Design review of the part built by this model. Coordinates are the model's own, in mm. A direction names the side the tool comes from. Give positions to 0.01 mm unless a question says otherwise; leave off trailing zeros. Loops run counter-clockwise (first coordinate to the right, second up) from the corner with the lowest first, then second, coordinate; pieces in that order, holes last. Notation, with made-up numbers: (37.25, 61.5) -> (87.25, 61.5) arc R33 cw to (87.25, 90.5) -> close; hole circle Ø7 at (86.25, -13.75). An arc over 180 degrees is marked (long way). Use a Markdown table: item, result. Add a question column.
1. For pin 1 Ø12 at (x, y) = (-92.5, 55.5) entering from -Z; pin 2 Ø11 at (y, z) = (56.5, 20) entering from -X; pin 3 Ø10 at (x, z) = (-135, 12.5) entering from +Y; pin 4 Ø3.5 at (x, z) = (-165.5, 38) entering from -Y, all flat-tipped, find the tip position at first contact; note any pin that passes through.
2. For faces 1 (the flat face through (-128.08, 5.65, 1.48)), 2 (the flat face through (-78.222, 44, 2)), 3 (the flat face through (-168, 16.67, 38)), 4 (the flat face through (-178.222, 54, 20)), 5 (the flat face through (-128, 53.67, 20)), list the 3-axis set-ups (+Z, -Z, +X, -X, +Y, -Y) from which the entire face can be reached by the end or side of a thin tool; tool diameter is ignored.
3. Add section A-A (y = 13). State the section outline as (x, z) points, and give its area (3 significant figures).
4. Add section B-B (y = 48.5). State the section outline as (x, z) points, and give its area (3 significant figures).
5. Add section D-D (x = -165). State the section outline as (y, z) points.
6. To check wall thickness, follow line 1 (Z direction, x = -99, y = 29); line 2 (Y direction, x = -147, z = 8); line 3 (X direction, y = 30, z = 38). State the ranges of each line that lie inside material, in increasing order.
7. Draft analysis for pull direction Z (two halves, no side actions). For faces 6 (the flat face through (-124, 38, 0)), 7 (the flat face through (-129, 62, 3)), 8 (the flat face through (-135, 39, 40)), 9 (the flat face through (-88.08, 5.65, 38.48)), state which applies: pulls with the +Z half, pulls with the -Z half, needs draft (parallel to the pull), parting line crosses it, or undercut.
8. Add section C-C (z = 12.5). State the section outline as (x, y) points.
```python
from build123d import *

# Parameters (mm, degrees)
F0_R      = 5
F1_DEPTH  = 40
F5_W      = 100
F5_H      = 3
F6_DEPTH  = 28
F7_W      = 100
F7_H      = 3
F8_DEPTH  = 10
F7_H_2    = 40
F13_DEPTH = 116.001
F14_W     = 100
F14_H     = 3
F15_DEPTH = 10
F18_DEPTH = 40.001
F19_SIZE  = 2
F20_SIZE  = 2
F21_W     = 67.4691606036
F21_H     = 7
F22_DEPTH = 116.001


with BuildPart() as f1:
    # F0 (on Top) → F1 (new body)
    with BuildSketch(Plane.XY):
        with BuildLine():
            Line((21.777506699, 52.6698508731), (21.777506699, 56.6698508731))
            Line((21.777506699, 56.6698508731), (-78.222493301, 56.6698508731))
            Line((-78.222493301, 56.6698508731), (-78.222493301, 16.6698508731))
            Line((-78.222493301, 16.6698508731), (-58.222493301, -5.6908289019))
            Line((-58.222493301, -5.6908289019), (-38.222493301, 16.6698508731))
            Line((-38.222493301, 16.6698508731), (-18.222493301, -5.6908289019))
            Line((-18.222493301, -5.6908289019), (1.777506699, 16.6698508731))
            Line((1.777506699, 16.6698508731), (21.777506699, 16.6698508731))
            Line((21.777506699, 16.6698508731), (31.377506699, 23.8698508731))
            ThreePointArc((31.377506699, 23.8698508731), (36.9564394679, 41.7294951294), (21.777506699, 52.6698508731))
        make_face()
        with Locations((21.777506699, 36.6698508731)):
            Circle(F0_R, mode=Mode.SUBTRACT)
    extrude(amount=F1_DEPTH)


with BuildPart() as f2_1:
    # F2: copy of F1
    add(f1.part.moved(Location((0, 0, 28))))


with BuildPart() as f4_1:
    # F4: copy of F1
    add(f1.part.moved(Location((0, 0, 34))))


with BuildPart() as f6:
    # F5 (on face) → F6 (new body)
    with BuildSketch(Plane.XY.offset(40)):
        with Locations((-28.222493301, 55.1698508731)):
            Rectangle(F5_W, F5_H)
    extrude(amount=F6_DEPTH)


with BuildPart() as f8:
    # F7 (on face) → F8 (new body)
    with BuildSketch(Plane(origin=(0, 56.6698508731, 0), x_dir=(-1, 0, 0), z_dir=(0, 1, 0))):
        with Locations((28.222493301, 69.5)):
            Rectangle(F7_W, F7_H)
    extrude(amount=F8_DEPTH)


with BuildPart() as f8b:
    # F7 (on face) → F8, piece 2 (new body)
    with BuildSketch(Plane(origin=(0, 56.6698508731, 0), x_dir=(-1, 0, 0), z_dir=(0, 1, 0))):
        with Locations((28.222493301, 20)):
            Rectangle(F7_W, F7_H_2)
    extrude(amount=F8_DEPTH)


with BuildPart() as f1_1:
    add(f1.part)

    # F12 (on face) → F13 (cut, through all)
    with BuildSketch(Plane(origin=(-78.222493301, 0, 0), x_dir=(0, -1, 0), z_dir=(-1, 0, 0))):
        Polygon((15.5293103307, 30), (-53.6698508731, 30), (-53.6698508731, 3), (13.7041052803, 3), align=None)
    extrude(amount=-F13_DEPTH, mode=Mode.SUBTRACT)

    # F14 (on face) → F15 (join)
    with BuildSketch(Plane(origin=(0, 56.6698508731, 0), x_dir=(-1, 0, 0), z_dir=(0, 1, 0))):
        with Locations((28.222493301, 1.5)):
            Rectangle(F14_W, F14_H)
        with Locations((28.222493301, 38.5)):
            Rectangle(F14_W, F14_H)
    extrude(amount=F15_DEPTH)

    # F16: F1 across face


with BuildPart() as f1_2:
    add(f1_1.part)
    add(f1_1.part.mirror(Plane(origin=(-78.222493301, 41.2061594964, 25.2897125567), x_dir=(0, -1, 0), z_dir=(-1, 0, 0))))

    # F17 (on face) → F18 (cut, through all)
    with BuildSketch(Plane.XY.offset(40)):
        Polygon((-78.222493301, 86.7001339793), (-78.222493301, 16.6698508731), (-78.222493301, -27.7220606804), (68.2113543153, -27.7220606804), (68.2113543153, 86.7001339793), align=None)
    extrude(amount=-F18_DEPTH, mode=Mode.SUBTRACT)

    # F19
    f19_edges = [f1_2.edges().sort_by_distance(p)[0] for p in [
        (-178.222493, 56.669851, 20),
    ]]
    chamfer(f19_edges, length=F19_SIZE)

    # F20
    f20_edges = [f1_2.edges().sort_by_distance(p)[0] for p in [
        (-78.222493, 56.669851, 20),
    ]]
    chamfer(f20_edges, length=F20_SIZE)

    # F21 (on face) → F22 (cut, through all)
    with BuildSketch(Plane.YZ.offset(-78.222493301)):
        with Locations((19.9352705713, 33.5)):
            Rectangle(F21_W, F21_H)
    extrude(amount=-F22_DEPTH, mode=Mode.SUBTRACT)


solid = f1_2.part
```
Taken from the geometry:
| question | item | result |
|---|---|---|
| 1 | pin 1 | stops at z = 0 |
| 1 | pin 2 | stops at x = -178.22 |
| 1 | pin 3 | stops at y = 56.67 |
| 1 | pin 4 | stops at y = 16.67 |
| 2 | face 1 | +Z, -Z, -Y |
| 2 | face 2 | +Z, -Z, +X, +Y, -Y |
| 2 | face 3 | +Z, -Z, -X, -Y |
| 2 | face 4 | +Z, -Z, -X, +Y |
| 2 | face 5 | +X, -X, -Y |
| 3 | outline | (-154.94, 0) -> (-121.5, 0) -> (-121.5, 3) -> (-154.94, 3) -> close; (-154.94, 37) -> (-121.5, 37) -> (-121.5, 40) -> (-154.94, 40) -> close; (-114.94, 0) -> (-81.5, 0) -> (-81.5, 3) -> (-114.94, 3) -> close; (-114.94, 37) -> (-81.5, 37) -> (-81.5, 40) -> (-114.94, 40) -> close |
| 3 | area | 401 mm^2 |
| 4 | outline | (-189, 0) -> (-78.22, 0) -> (-78.22, 3) -> (-189, 3) -> close; (-189, 37) -> (-78.22, 37) -> (-78.22, 40) -> (-189, 40) -> close |
| 4 | area | 665 mm^2 |
| 5 | outline | (16.67, 0) -> (66.67, 0) -> (66.67, 3) -> (56.67, 3) -> (56.67, 37) -> (66.67, 37) -> (66.67, 40) -> (16.67, 40) -> (16.67, 37) -> (53.67, 37) -> (53.67, 3) -> (16.67, 3) -> close |
| 6 | line 1 | z = 0 to 3, 37 to 40 |
| 6 | line 2 | y = 53.67 to 56.67 |
| 6 | line 3 | x = -192.77 to -78.22 |
| 7 | face 6 | pulls with the -Z half |
| 7 | face 7 | undercut |
| 7 | face 8 | pulls with the +Z half |
| 7 | face 9 | needs draft |
| 8 | outline | (-178.22, 53.67) -> (-78.22, 53.67) -> (-78.22, 54.67) -> (-80.22, 56.67) -> (-176.22, 56.67) -> (-178.22, 54.67) -> close |
